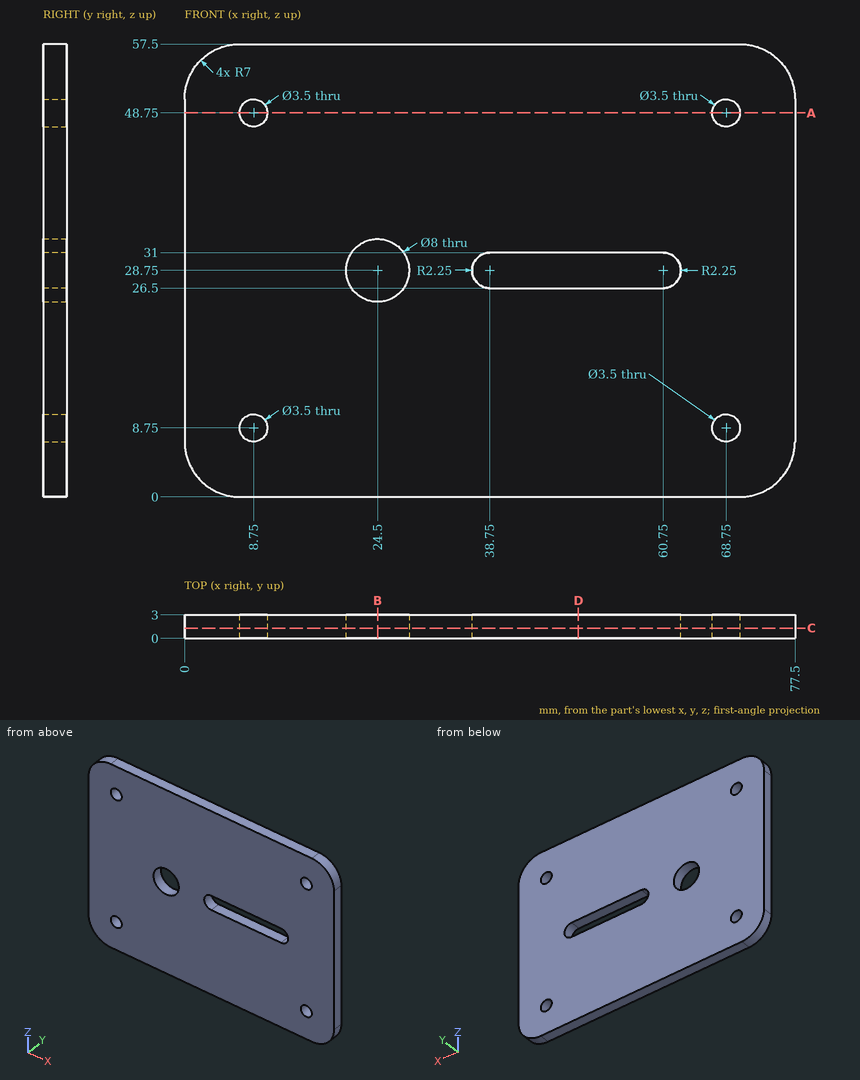
Here's the drawing with two shaded views (mm, measured from the low corner). I have some questions. Give positions to 0.01 mm unless a question says otherwise; leave off trailing zeros. Write each loop counter-clockwise with the first axis right and the second up, starting at its lowest first coordinate (ties: lowest second). Pieces come first, ordered by that corner, then holes. Notation, with made-up numbers: (-8, -35) -> (40, -35) arc R21 ccw to (40, -21) -> close; hole circle Ø1 at (-2.75, 10). An arc over 180 degrees is marked (long way). Answer as a JSON object with one key per item and string values. Group by question number.
Item 1: I'm going to push a flat-ended pin straight in: P1, Ø5, axis at x = 24.5, z = 28.75, coming from the +Y side. Where does the tip first touch, or does it pass through?
Item 2: Suppose I cut it at D-D (x = 50). Please give me the cut outline in (y, z), plus the area to 3 significant figures.
Item 3: Suppose I cut it at B-B (x = 24.5). Please give me the cut outline in (y, z).
Item 4: Suppose I cut it at C-C (y = 1.3). Please give me the cut outline in (x, z).
Item 5: Suppose I cut it at A-A (z = 48.75). Please give me the cut outline in (x, y), plus the area to 4 significant figures.
Item 6: Please list where these lines run through material, in increasing order: line 1 (Z direction, x = 8.75, y = 1.2); line 2 (X direction, y = 2.2, z = 8.75); line 3 (Z direction, x = 60.5, y = 0.7). Write a range as [from, to].
Findings:
{
 "1": {"P1": "passes through"},
 "2": {"outline": "(0, 0) -> (3, 0) -> (3, 26.5) -> (0, 26.5) -> close; (0, 31) -> (3, 31) -> (3, 57.5) -> (0, 57.5) -> close", "area": "159 mm²"},
 "3": {"outline": "(0, 0) -> (3, 0) -> (3, 24.75) -> (0, 24.75) -> close; (0, 32.75) -> (3, 32.75) -> (3, 57.5) -> (0, 57.5) -> close"},
 "4": {"outline": "(0, 7) arc R7 ccw to (7, 0) -> (70.5, 0) arc R7 ccw to (77.5, 7) -> (77.5, 50.5) arc R7 ccw to (70.5, 57.5) -> (7, 57.5) arc R7 ccw to (0, 50.5) -> close; hole circle Ø3.5 at (8.75, 8.75); hole circle Ø3.5 at (8.75, 48.75); hole circle Ø8 at (24.5, 28.75); hole (38.75, 26.5) -> (60.75, 26.5) arc R2.25 ccw to (60.75, 31) -> (38.75, 31) arc R2.25 ccw to start; hole circle Ø3.5 at (68.75, 8.75); hole circle Ø3.5 at (68.75, 48.75)"},
 "5": {"outline": "(0, 0) -> (7, 0) -> (7, 3) -> (0, 3) -> close; (10.5, 0) -> (67, 0) -> (67, 3) -> (10.5, 3) -> close; (70.5, 0) -> (77.5, 0) -> (77.5, 3) -> (70.5, 3) -> close", "area": "211.5 mm²"},
 "6": {"line 1": "z = [0, 7], [10.5, 47], [50.5, 57.5]", "line 2": "x = [0, 7], [10.5, 67], [70.5, 77.5]", "line 3": "z = [0, 26.5], [31, 57.5]"}
}
